Part model, mm, in its own coordinate system. A direction names the side the tool comes from. Coordinates: 2 decimals unless noted, no trailing zeros. Write each loop counter-clockwise with the first axis right and the second up, starting at its lowest first coordinate (ties: lowest second). Pieces come first, ordered by that corner, then holes. Notation, with made-up numbers: M 8,19.25 L 21,19.25 A21 cw 21,23.25 Z; hole C 49.25,48 d3. An arc over 180 degrees is marked long. Use a Markdown table: item, result. Add a question column.
Q1. Slice it at C-C on z = -68.5. Write the cut outline in (x, y), then the cut area to 3 significant figures.
Q2. Slice it at B-B on z = -190.5. Write the cut outline in (x, y) (1 decimal), then the cut area to 3 significant figures.
Q3. Mould opens along X. For faces 3 (the flat face through (25.4, 13, -150)), 4 (the cylindrical face through (0.78, 14.63, -238.78)), 5 (the cylindrical face through (15.5, 0.8, -11.2)) say: released by +X, released by -X, zero draft, split by the parting line, or undercut.
Q4. Pin check, flat tip, straight feed: pin 1 Ø4 at (y, z) = (12.7, -266.7) entering from +X. Stop position of the tip, or through.
Q5. Wall check: L1, parallel to X at y = 0.8, z = -12.7 (3 decimals); L2, parallel to X at y = 1.75, z = -90. Give the ranges that are in metal, low to high. Write a range as from..to.
Q6. Tool access for faces 1 (the cylindrical face through (24.6, 14.63, -238.78)), 2 (the flat face through (1.588, 13, -150)): list every direction of +Z, -Z, +X, -X, +Y, -Y with a clear straight run to the whole face (end or side of a thin tool).
Q7. Slice it at A-A on y = 6. Write the cut outline in (x, z).
Autodesk Inventor part; units mm, degrees
ref_plane "YZ Plane" through (0, 0, 0) normal (1, 0, 0) x (0, 1, 0)
ref_plane "XZ Plane" through (0, 0, 0) normal (0, 1, 0) x (-1, 0, 0)
ref_plane "XY Plane" through (0, 0, 0) normal (0, 0, 1) x (1, 0, 0)
sketch "Sketch1" plane through (0, 0, 0) normal (0, 0, 1) x (1, 0, 0)
  line L0 (0, 0) -> (25.4, 0)
  line L1 (25.4, 0) -> (25.4, 25.4)
  line L2 (25.4, 25.4) -> (0, 25.4)
  line L3 (0, 25.4) -> (0, 0)
  line L4 (1.5875, 23.8125) -> (23.8125, 23.8125)
  line L5 (23.8125, 23.8125) -> (23.8125, 1.5875)
  line L6 (23.8125, 1.5875) -> (1.5875, 1.5875)
  line L7 (1.5875, 1.5875) -> (1.5875, 23.8125)
  dimension "d0" = 25.4
  dimension "d1" = 25.4
  dimension "d2" = 1.5875
extrude "Extrusion1" add sketch "Sketch1" against normal blind 304.8
sketch "Sketch2" plane through (0, 25.4, 0) normal (0, 1, 0) x (1, 0, 0)
  line L0 (25.4, 0) -> (0, 0)
  point P0 (12.7, 12.7)
  point P1 (12.7, 50.8)
  dimension "d5" = 12.7
  dimension "d6" = 38.1
hole "Hole1" at (12.7, 25.4, -12.7) at (12.7, 25.4, -50.8) direction (0, -1, 0) diameter 6.35 depth 25.4 tip angle 118
sketch "Sketch3" plane through (25.4, 0, 0) normal (1, 0, 0) x (0, 0, -1)
  line L0 (304.8, 0) -> (304.8, 25.4)
  point P0 (292.1, 12.7)
  point P1 (266.7, 12.7)
  point P2 (241.3, 12.7)
  point P3 (215.9, 12.7)
  point P4 (190.5, 12.7)
  point P5 (165.1, 12.7)
  dimension "d14" = 25.4
  dimension "d15" = 25.4
  dimension "d16" = 25.4
  dimension "d17" = 25.4
  dimension "d18" = 12.7
  dimension "d26" = 25.4
hole "Hole2" at (25.4, 12.7, -292.1) at (25.4, 12.7, -266.7) at (25.4, 12.7, -241.3) at (25.4, 12.7, -215.9) at (25.4, 12.7, -190.5) at (25.4, 12.7, -165.1) direction (-1, 0, 0) diameter 6.35 depth 25.4 tip angle 118
properties part number "1tube_10_framegrabberarm"
Recorded:
| question | item | result |
|---|---|---|
| 1 | outline | M 0,0 L 25.4,0 L 25.4,25.4 L 0,25.4 Z; hole M 1.59,1.59 L 23.81,1.59 L 23.81,23.81 L 1.59,23.81 Z |
| 1 | area | 151 mm² |
| 2 | outline | M 0,0 L 25.4,0 L 25.4,9.5 L 23.8,9.5 L 23.8,1.6 L 1.6,1.6 L 1.6,9.5 L 0,9.5 Z; M 0,15.9 L 1.6,15.9 L 1.6,23.8 L 23.8,23.8 L 23.8,15.9 L 25.4,15.9 L 25.4,25.4 L 0,25.4 Z |
| 2 | area | 131 mm² |
| 3 | face 3 | released by +X |
| 3 | face 4 | zero draft |
| 3 | face 5 | undercut |
| 4 | pin 1 | through |
| 5 | L1 | 0..9.525, 15.875..25.4 |
| 5 | L2 | 0..1.59, 23.81..25.4 |
| 6 | face 1 | +X, -X |
| 6 | face 2 | +Z, -Z |
| 7 | outline | M 0,-304.8 L 1.59,-304.8 L 1.59,0 L 0,0 Z; M 23.81,-304.8 L 25.4,-304.8 L 25.4,0 L 23.81,0 Z |
